from build123d import *

# Parameters (mm, degrees)
F0_R     = 4.7625
F2_DEPTH = 3.175
F3_R     = 2.54


# Not quite as in the source:
# - a variable given as a bare number and used for a length is read in inches; the dataset says mm whatever the document's units were


with BuildPart() as f2:
    # F0 (on Top) → F2 (new body, symmetric)
    with BuildSketch(Plane.XY):
        with BuildLine():
            Line((-203.2, 0), (0, 0))
            Line((0, 0), (0, 19.05))
            Line((0, 19.05), (-203.2, 19.05))
            ThreePointArc((-203.2, 19.05), (-212.725, 9.525), (-203.2, 0))
        make_face()
        with Locations((-203.2, 9.525)):
            Circle(F0_R, mode=Mode.SUBTRACT)
    extrude(amount=F2_DEPTH, both=True)

    # F3
    f3_edges = [f2.edges().sort_by_distance(p)[0] for p in [
        (-101.6, 0, 3.175),
        (-101.6, 0, -3.175),
    ]]
    fillet(f3_edges, radius=F3_R)


solid = f2.part
The model under review builds one solid part; all positions refer to its coordinate system, in mm. Give positions to 0.01 mm unless a question says otherwise; leave off trailing zeros. Loops run counter-clockwise (first coordinate to the right, second up) from the corner with the lowest first, then second, coordinate; pieces in that order, holes last. Notation, with made-up numbers: (-29.75, 8) -> (-23.75, 8) arc R18 cw to (-23.75, 39) -> close; hole circle Ø5 at (21.25, 66.25). An arc over 180 degrees is marked (long way). Put each result on its own line as item: value. Start each with the question number.
1. We need section A-A on x = -183.5. State the section outline as (y, z) points (3 decimals).
2. Clearance check with a flat-ended pin moving along its axis: P1, Ø8.5, axis at x = -203.2, y = 9.525, coming from the +Z side. State where the tip first meets the part, or that it passes through.
3. Wall thickness on probe 1 along Y at (x, z) = (-203.2, 0.75); probe 2 along X at (y, z) = (11.5, 0); probe 3 along Y at (x, z) = (-203.2, -1.5): over which ranges is each line inside the solid? List them lowest first.
4. We need section B-B on z = 1.75. State the section outline as (x, y) points (1 decimal).
Determined:
1. outline: (0, -0.635) arc R2.54 ccw to (2.54, -3.175) -> (16.51, -3.175) arc R2.54 ccw to (19.05, -0.635) -> (19.05, 0.635) arc R2.54 ccw to (16.51, 3.175) -> (2.54, 3.175) arc R2.54 ccw to (0, 0.635) -> close
2. P1: through
3. probe 1: 0 to 4.76, 14.29 to 19.05
3. probe 2: -212.52 to -207.53, -198.87 to 0
3. probe 3: 0.15 to 4.76, 14.29 to 18.9
4. outline: (-203.2, 0.3) -> (0, 0.3) -> (0, 18.8) -> (-203.2, 18.8) arc R9.3 ccw to start; hole circle Ø9.5 at (-203.2, 9.5)
